Work out the finished part from the listing and answer in its coordinate system (mm). Round coordinates to 2 decimals unless told otherwise and drop trailing zeros. Order: outer loops, then holes, each group sorted by start corner. A loop starts at its lowest first (then second) coordinate and runs counter-clockwise, first axis right, second up. Notation, with made-up numbers: M 82.5,17.25 L 113.5,17.25 A19 cw 113.5,31.25 Z; hole C -12.75,74.25 d10. An arc over 180 degrees is marked long. Return JSON: item names as keys, results as strings.
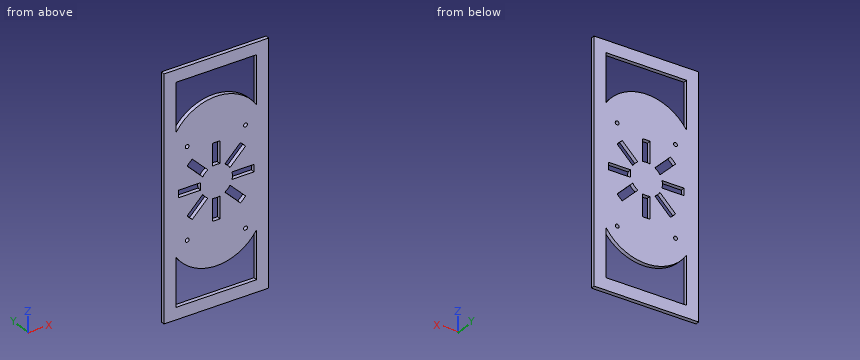
Autodesk Inventor part; units mm, degrees
ref_plane "Work Plane1" through (0, 0, -100) normal (0, 0, -1) x (-1, 0, 0)
ref_plane "YZ Plane" through (0, 0, 0) normal (1, 0, 0) x (0, 1, 0)
ref_plane "XZ Plane" through (0, 0, 0) normal (0, 1, 0) x (-1, 0, 0)
sketch "Boceto1" plane through (0, 0, 0) normal (0, 1, 0) x (-1, 0, 0)
  line L0 (0, 0) -> (86.6, 0)
  line L1 (86.6, 0) -> (86.6, -200)
  line L2 (86.6, -200) -> (0, -200)
  line L3 (0, -200) -> (0, 0)
  dimension "d0" = 200
  dimension "d1" = 86.6
extrude "Extrusión1" add sketch "Boceto1" along normal blind 3.3
sketch "Boceto2" plane through (0, 3.3, 0) normal (0, 1, 0) x (1, 0, 0)
  circle A0 centre (-43.3, 100) radius 13.3 construction
  circle A1 centre (-43.3, 100) radius 31.3 construction
  line L0 (-86.6, 0) -> (0, 0)
  line L1 (0, 0) -> (0, 200)
  line L2 (0, 200) -> (-86.6, 200)
  line L3 (-86.6, 200) -> (-86.6, 0)
  line L4 (0, 200) -> (-86.6, 200)
  line L5 (-46.3, 68.8441) -> (-46.3, 87.0428)
  line L6 (-40.3, 68.8441) -> (-40.3, 87.0428)
  arc A2 (-46.3, 87.0428) -> (-40.3, 87.0428) centre (-43.3, 100) ccw
  arc A3 (-46.3, 68.8441) -> (-40.3, 68.8441) centre (-43.3, 100) ccw
  line L7 (-19.1481, 80.0908) -> (-32.0165, 92.9592)
  arc A4 (-23.3908, 75.8481) -> (-19.1481, 80.0908) centre (-43.3, 100) ccw
  line L8 (-23.3908, 75.8481) -> (-36.2592, 88.7165)
  arc A5 (-36.2592, 88.7165) -> (-32.0165, 92.9592) centre (-43.3, 100) ccw
  line L9 (-12.1441, 103) -> (-30.3428, 103)
  arc A6 (-12.1441, 97) -> (-12.1441, 103) centre (-43.3, 100) ccw
  line L10 (-12.1441, 97) -> (-30.3428, 97)
  arc A7 (-30.3428, 97) -> (-30.3428, 103) centre (-43.3, 100) ccw
  line L11 (-23.3908, 124.1519) -> (-36.2592, 111.2835)
  arc A8 (-19.1481, 119.9092) -> (-23.3908, 124.1519) centre (-43.3, 100) ccw
  line L12 (-19.1481, 119.9092) -> (-32.0165, 107.0408)
  arc A9 (-32.0165, 107.0408) -> (-36.2592, 111.2835) centre (-43.3, 100) ccw
  line L13 (-46.3, 131.1559) -> (-46.3, 112.9572)
  arc A10 (-40.3, 131.1559) -> (-46.3, 131.1559) centre (-43.3, 100) ccw
  line L14 (-40.3, 131.1559) -> (-40.3, 112.9572)
  arc A11 (-40.3, 112.9572) -> (-46.3, 112.9572) centre (-43.3, 100) ccw
  line L15 (-67.4519, 119.9092) -> (-54.5835, 107.0408)
  arc A12 (-63.2092, 124.1519) -> (-67.4519, 119.9092) centre (-43.3, 100) ccw
  line L16 (-63.2092, 124.1519) -> (-50.3408, 111.2835)
  arc A13 (-50.3408, 111.2835) -> (-54.5835, 107.0408) centre (-43.3, 100) ccw
  line L17 (-74.4559, 97) -> (-56.2572, 97)
  arc A14 (-74.4559, 103) -> (-74.4559, 97) centre (-43.3, 100) ccw
  line L18 (-74.4559, 103) -> (-56.2572, 103)
  arc A15 (-56.2572, 103) -> (-56.2572, 97) centre (-43.3, 100) ccw
  line L19 (-63.2092, 75.8481) -> (-50.3408, 88.7165)
  arc A16 (-67.4519, 80.0908) -> (-63.2092, 75.8481) centre (-43.3, 100) ccw
  line L20 (-67.4519, 80.0908) -> (-54.5835, 92.9592)
  arc A17 (-54.5835, 92.9592) -> (-50.3408, 88.7165) centre (-43.3, 100) ccw
  line L21 (-86.6, 200) -> (-86.6, 0)
  line L22 (0, 0) -> (0, 200)
  point P0 (-43.3, 200)
  point P1 (-86.6, 100)
  point P2 (-43.3, 200)
  point P3 (-43.3, 86.7)
  point P4 (-33.8955, 90.5955)
  point P5 (-30, 100)
  point P6 (-33.8955, 109.4045)
  point P7 (-43.3, 113.3)
  point P8 (-52.7045, 109.4045)
  point P9 (-56.6, 100)
  point P10 (-52.7045, 90.5955)
  dimension "d10" = 18
  dimension "d11" = 6
  dimension "d14" = 360
  dimension "d19" = 30
extrude "Extrusión2" cut sketch "Boceto2" against normal blind 10 contours L5 A2 L6 A3 | A4 L8 A5 L7 | A6 L10 A7 L9 | A8 L12 A9 L11 | A10 L14 A11 L13 | A12 L16 A13 L15 | A14 L18 A15 L17 | A16 L20 A17 L19
sketch "Sketch3" plane through (0, 3.3, 0) normal (0, 1, 0) x (1, 0, 0)
  line L0 (-86.6, 200) -> (-86.6, 0)
  line L1 (-69.975, 150.795) -> (-16.625, 150.795) construction
  line L2 (-16.625, 150.795) -> (-16.625, 49.205) construction
  line L3 (-16.625, 49.205) -> (-69.975, 49.205) construction
  line L4 (-69.975, 49.205) -> (-69.975, 150.795) construction
  line L5 (0, 200) -> (-86.6, 200)
  circle A0 centre (-67.425, 64.445) radius 1.5875
  circle A1 centre (-19.165, 63.175) radius 1.5875
  circle A2 centre (-19.165, 145.725) radius 1.5875
  circle A3 centre (-67.425, 139.375) radius 1.5875
  circle A4 centre (-24.245, 115.245) radius 1.5875
  point P0 (0, 0)
  dimension "d21" = 101.59
  dimension "d22" = 53.35
  dimension "d23" = 16.625
  dimension "d24" = 49.205
  dimension "d25" = 15.24
  dimension "d26" = 3.175
  dimension "d28" = 50.8
  dimension "d29" = 13.97
  dimension "d30" = 2.54
  dimension "d31" = 90.17
  dimension "d32" = 96.52
  dimension "d34" = 50.8
  dimension "d35" = 2.54
  dimension "d36" = 66.04
  dimension "d37" = 7.62
extrude "Extrusion3" cut sketch "Sketch3" against normal blind 10 contours A0 | A1 | A2 | A3
sketch "Sketch4" plane through (0, 3.3, 0) normal (0, 1, 0) x (1, 0, 0)
  line L0 (-10, 10) -> (-76.6, 10)
  line L1 (-76.6, 10) -> (-76.6, 50)
  line L2 (-10, 10) -> (-10, 50)
  arc A0 (-76.6, 50) -> (-10, 50) centre (-43.3, 72.161) ccw
  line L3 (-86.6, 0) -> (0, 0)
  line L4 (-86.6, 200) -> (-86.6, 0)
  line L5 (0, 0) -> (0, 200)
  dimension "d40" = 10
  dimension "d41" = 10
  dimension "d42" = 10
  dimension "d43" = 40
  dimension "d44" = 40
ref_plane "Work Plane1" through (0, 0, -100) normal (0, 0, -1) x (-1, 0, 0)
extrude "Extrusion4" cut sketch "Sketch4" against normal blind 10
mirror "Mirror1" about plane through (0, 0, -100) normal (0, 0, -1) of "Extrusion4"
equation "\"d0\" = largo_base"
equation "\"d10\" = 1.5 * d4"
equation "\"d11\" = 0.2 * d19"
equation "\"d24\" = 0.5 * largo_base - 0.5 * d21"
equation "\"d34\" = d28"
equation "\"d35\" = d30"
equation "\"ancho_base\" = 80"
properties part number "Cuerpo - Base" material "ABS Plastic"
Item 1: Find section C-C (z = -116). Determine the outline of the cut face in (x, y), plus the area to 3 significant figures.
Output:
{"outline": "M -86.6,0 L -63.54,0 L -63.54,3.3 L -86.6,3.3 Z; M -55.06,0 L -46.3,0 L -46.3,3.3 L -55.06,3.3 Z; M -40.3,0 L -31.54,0 L -31.54,3.3 L -40.3,3.3 Z; M -23.06,0 L 0,0 L 0,3.3 L -23.06,3.3 Z", "area": "210 mm^2"}
Item 2: Find section D-D (z = -34). Determine the outline of the cut face in (x, y), plus the area to 3 significant figures.
Output:
{"outline": "M -86.6,0 L -76.6,0 L -76.6,3.3 L -86.6,3.3 Z; M -55.29,0 L -31.31,0 L -31.31,3.3 L -55.29,3.3 Z; M -10,0 L 0,0 L 0,3.3 L -10,3.3 Z", "area": "145 mm^2"}
Item 3: Find section A-A (z = -170). Determine the outline of the cut face in (x, y).
Output:
{"outline": "M -86.6,0 L -76.6,0 L -76.6,3.3 L -86.6,3.3 Z; M -10,0 L 0,0 L 0,3.3 L -10,3.3 Z"}
Item 4: Consider line 1 along Z through (x, y) = (-39, 0.95); line 2 along Z through (x, y) = (-29.5, 0.2); line 3 along Z through (x, y) = (-71.5, 0.85). Determine where each line is inside the solid, lowest interval first. Write a range as [from, to].
Output:
{"line 1": "z = [-200, -190], [-167.61, -32.39], [-10, 0]", "line 2": "z = [-200, -190], [-165.38, -118.04], [-109.56, -103], [-97, -90.44], [-81.96, -34.62], [-10, 0]", "line 3": "z = [-200, -190], [-156.21, -103], [-97, -43.79], [-10, 0]"}
Item 5: Find section B-B (x = -71). Determine the outline of the cut face in (y, z).
Output:
{"outline": "M 0,-200 L 3.3,-200 L 3.3,-190 L 0,-190 Z; M 0,-156.7 L 3.3,-156.7 L 3.3,-103 L 0,-103 Z; M 0,-97 L 3.3,-97 L 3.3,-43.3 L 0,-43.3 Z; M 0,-10 L 3.3,-10 L 3.3,0 L 0,0 Z"}
